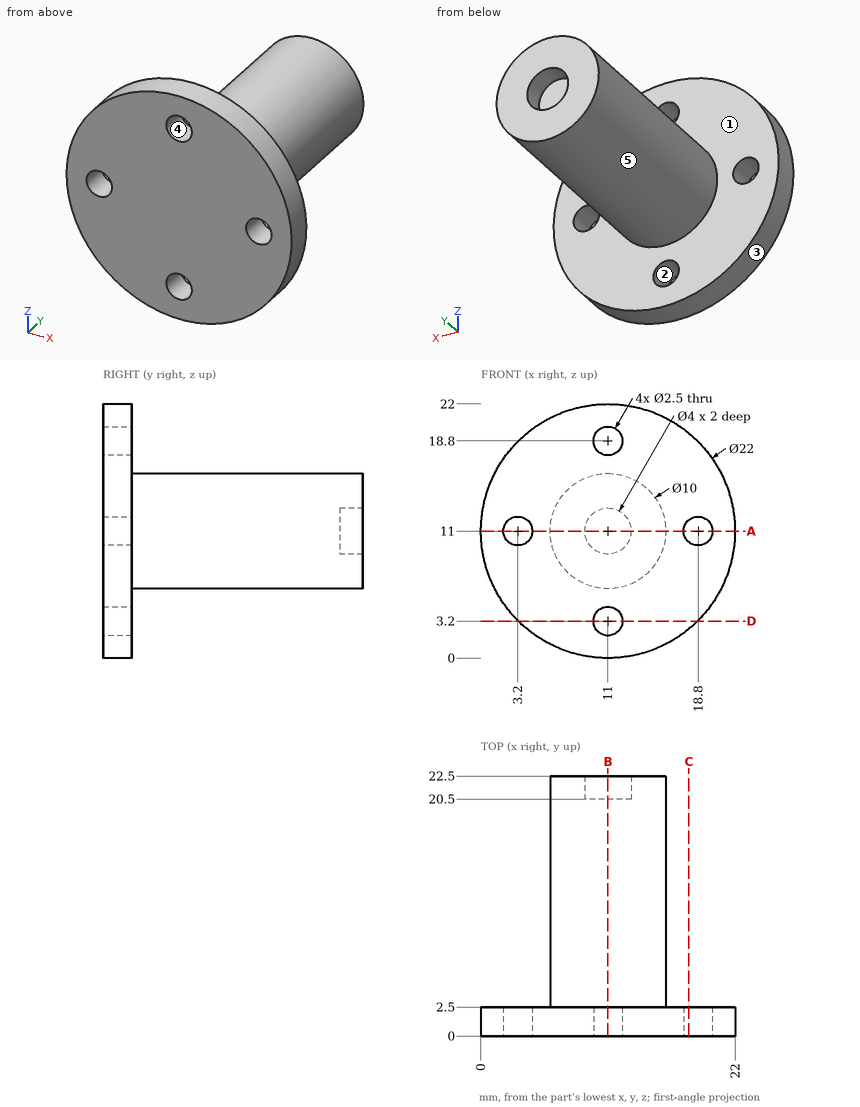
Here's the drawing with two shaded views (mm, measured from the low corner). I have some questions. A direction names the side the tool comes from. Round coordinates to 2 decimals unless told otherwise and drop trailing zeros. Loops run counter-clockwise (first coordinate to the right, second up) from the corner with the lowest first, then second, coordinate; pieces in that order, holes last. Notation, with made-up numbers: M 0.5,86 L 52.5,86 A7 ccw 52.5,96 Z; hole C -36.75,12 d4. An arc over 180 degrees is marked long. Answer as CSV lines item,"result".
1) Imagine slicing it at B-B on x = 11. List the corners of the cut face in (y, z) for me, and give its area (4 significant figures).
From the geometry:
outline,"M 0,0 L 2.5,0 L 2.5,1.95 L 0,1.95 Z; M 0,4.45 L 2.5,4.45 L 2.5,6 L 22.5,6 L 22.5,9 L 20.5,9 L 20.5,13 L 22.5,13 L 22.5,16 L 2.5,16 L 2.5,17.55 L 0,17.55 Z; M 0,20.05 L 2.5,20.05 L 2.5,22 L 0,22 Z"
area,"234.5 mm^2"
2) We'd pull the mould along X, two halves only. Please class the marked faces 1, 2 and 3: released by +X, released by -X, zero draft, split by the parting line, or undercut.
From the geometry:
face 1,"zero draft"
face 2,"undercut"
face 3,"split by the parting line"
3) Which directions (+Z, -Z, +X, -X, +Y, -Y) give clear straight access to the entire face, cutting with the end or side of a thin tool? Please do the marked faces 4 and 5.
From the geometry:
face 4,"+Y, -Y"
face 5,"+Y"
4) Imagine slicing it at C-C on x = 18. List the corners of the cut face in (y, z) for me, and give its area (3 significant figures).
From the geometry:
outline,"M 0,2.51 L 2.5,2.51 L 2.5,10.04 L 0,10.04 Z; M 0,11.96 L 2.5,11.96 L 2.5,19.49 L 0,19.49 Z"
area,"37.6 mm^2"
5) Imagine slicing it at D-D on z = 3.2. List the corners of the cut face in (x, y) for me, and give its area (3 significant figures).
From the geometry:
outline,"M 3.24,0 L 9.75,0 L 9.75,2.5 L 3.24,2.5 Z; M 12.25,0 L 18.76,0 L 18.76,2.5 L 12.25,2.5 Z"
area,"32.5 mm^2"
6) Imagine slicing it at A-A on z = 11. List the corners of the cut face in (x, y) for me.
From the geometry:
outline,"M 0,0 L 1.95,0 L 1.95,2.5 L 0,2.5 Z; M 4.45,0 L 17.55,0 L 17.55,2.5 L 16,2.5 L 16,22.5 L 13,22.5 L 13,20.5 L 9,20.5 L 9,22.5 L 6,22.5 L 6,2.5 L 4.45,2.5 Z; M 20.05,0 L 22,0 L 22,2.5 L 20.05,2.5 Z"
7) For pin 1 Ø5 at (y, z) = (9, 17) entering from -X; pin 2 Ø4 at (x, z) = (18.8, 11) entering from +Y; pin 3 Ø1.5 at (x, z) = (11, 18.8) entering from -Y; pin 4 Ø2 at (x, z) = (11.5, 11.5) entering from +Y, each with a flat end and sliding along its axis, tell me the tip position at first contact or that it passes through.
From the geometry:
pin 1,"x = 7.43"
pin 2,"y = 2.5"
pin 3,"through"
pin 4,"y = 20.5"
8) If I drill on probe 1 along X at (y, z) = (1.65, 11); probe 2 along X at (y, z) = (1.25, 12); probe 3 along X at (y, z) = (21.2, 11), over which ranges is the centre line in solid material (lowest first)?
From the geometry:
probe 1,"0 to 1.95, 4.45 to 17.55, 20.05 to 22"
probe 2,"0.05 to 2.45, 3.95 to 18.05, 19.55 to 21.95"
probe 3,"6 to 9, 13 to 16"
